Source: CAD feature listing. Evaluate the final solid. Frame: model axes, mm. A direction names the side the tool comes from. Give positions to 0.01 mm unless a question says otherwise; leave off trailing zeros. Write each loop counter-clockwise with the first axis right and the second up, starting at its lowest first coordinate (ties: lowest second). Pieces come first, ordered by that corner, then holes. Notation, with made-up numbers: (-3, 77) -> (48, 77) arc R15 cw to (48, 90) -> close; hole circle Ø5 at (82, 68). An arc over 180 degrees is marked (long way). Use one line per item in the form item = value. Start each with the question number.
(1) Material intervals for line 1 along Y through (x, z) = (-2, 3); line 2 along Y through (x, z) = (-4.75, 12.5), sorted ascending. Write a range as from..to.
(2) Cut plane C-C, the plane z = 8.25. Output: boundary loops of the cut face in (x, y).
(3) Cut plane B-B, the plane x = -5.75. Output: boundary loops of the cut face in (y, z).
(4) Cut plane A-A, the plane z = 14.25. Output: boundary loops of the cut face in (x, y), and give its area (3 significant figures).
(5) Draft query along X for faces 1 (the face through (0, 8, 5)), 2 (the face through (0, 5, 8)), 3 (the face through (-7, 0, 14)). Return one class per face: pulls with the +X half, pulls with the -X half, needs draft (parallel to the pull), parting line crosses it, or undercut.
(6) First-contact query: P1, Ø3, axis at x = 6, y = -2.5, coming from the +Z side; P2, Ø8, axis at x = -0.5, y = -0.5, coming from the -Z side; P3, Ø3, axis at x = -0.5, z = 15, coming from the +Y side. Flat tips, straight axial feed; report the tip coordinate or a pass-through.
(7) Set-up query: faces 4 (the face through (-6, 0, 18)), 5 (the face through (7, 0, 14)), 6 (the face through (-5, 0, 8)), 7 (the face through (0, 7, 15)). Return all of +Z, -Z, +X, -X, +Y, -Y with unobstructed straight access to the full face (end or side cutting, diameter ignored); none if empty.
(8) Cut plane D-D, the plane y = 6.75. Output: boundary loops of the cut face in (x, z).
from build123d import *

# Parameters (mm, degrees)
BOX001_W      = 10
BOX001_H      = 10
BOX001_DEPTH  = 17
EXTRUDE_DEPTH = 14
BOX_W         = 16
BOX_H         = 16
BOX_DEPTH     = 10


with BuildPart() as cube001:
    # Box001 → Box001 (new body)
    with BuildSketch(Plane(origin=(-5, -5, 0), x_dir=(1, 0, 0), z_dir=(0, 0, 1))):
        with Locations((5, 5)):
            Rectangle(BOX001_W, BOX001_H)
    extrude(amount=BOX001_DEPTH)


with BuildPart() as extrude_body:
    # Sketch → Extrude (new body)
    with BuildSketch(Plane(origin=(-7, -7, 0), x_dir=(1, 0, 0), z_dir=(0, -1, 0))):
        with BuildLine():
            ThreePointArc((7, 19.039578), (4.192599, 19.937873), (1.971545, 18))
            Line((1.971545, 18), (0, 18))
            Line((0, 18), (0, 10))
            Line((0, 10), (14, 10))
            Line((14, 10), (14, 19))
            Line((14, 19), (11.183659, 19))
            ThreePointArc((11.183659, 19), (9.512524, 19.999072), (7.783659, 19.103606))
            ThreePointArc((7, 19.039578), (7.407388, 18.881168), (7.783659, 19.103606))
        make_face()
    extrude(amount=-EXTRUDE_DEPTH)


with BuildPart() as cut:
    # Box → Box (new body)
    with BuildSketch(Plane(origin=(-8, -8, 0), x_dir=(1, 0, 0), z_dir=(0, 0, 1))):
        with Locations((8, 8)):
            Rectangle(BOX_W, BOX_H)
    extrude(amount=BOX_DEPTH)

    # Fusion: union Extrude body
    add(extrude_body.part)

    # Cut: cut Cube001
    add(cube001.part, mode=Mode.SUBTRACT)


solid = cut.part
Geometry says:
q1.line_1 = -8..-5, 5..8
q1.line_2 = -7..-5, 5..7
q2.outline = (-8, -8) -> (8, -8) -> (8, 8) -> (-8, 8) -> close; hole (-5, -5) -> (5, -5) -> (5, 5) -> (-5, 5) -> close
q3.outline = (-8, 0) -> (8, 0) -> (8, 10) -> (7, 10) -> (7, 18) -> (-7, 18) -> (-7, 10) -> (-8, 10) -> close
q4.outline = (-7, -7) -> (7, -7) -> (7, 7) -> (-7, 7) -> close; hole (-5, -5) -> (5, -5) -> (5, 5) -> (-5, 5) -> close
q4.area = 96.0 mm^2
q5.face_1 = needs draft
q5.face_2 = undercut
q5.face_3 = pulls with the -X half
q6.P1 = 19
q6.P2 = 17
q6.P3 = 7
q7.face_4 = +Z, -X, +Y, -Y
q7.face_5 = +Z, +X, +Y, -Y
q7.face_6 = -Z
q7.face_7 = +Z, +X, -X, +Y
q8.outline = (-8, 0) -> (8, 0) -> (8, 10) -> (7, 10) -> (7, 19) -> (4.18, 19) arc R2 ccw to (0.78, 19.1) arc R0.5 cw to (0, 19.04) arc R3 ccw to (-5.03, 18) -> (-7, 18) -> (-7, 10) -> (-8, 10) -> close
